Source: CAD feature listing. Evaluate the final solid. Frame: model axes, mm. A direction names the side the tool comes from. Coordinates: 2 decimals unless noted, no trailing zeros. Order: outer loops, then holes, each group sorted by start corner. A loop starts at its lowest first (then second) coordinate and runs counter-clockwise, first axis right, second up. Notation, with made-up numbers: (-30.75, 36.5) -> (13.25, 36.5) arc R30 cw to (13.25, 61.5) -> close; hole circle Ø11 at (13, 41). An arc over 180 degrees is marked (long way). Put each result on its own line as item: value.
from build123d import *

# Parameters (mm, degrees)
F0_R     = 11
F0_R_2   = 4
F1_DEPTH = 5.5
F2_R     = 12.5
F2_R_2   = 4
F3_DEPTH = 1.5
F4_R     = 9
F4_R_2   = 6
F5_DEPTH = 0.2
F6_R     = 9
F6_R_2   = 6
F7_DEPTH = 0.2
F8_R     = 0.3


with BuildPart() as f1:
    # F0 (on Front) → F1 (new body)
    with BuildSketch(Plane.XZ):
        Circle(F0_R)
        Circle(F0_R_2, mode=Mode.SUBTRACT)
    extrude(amount=F1_DEPTH)

    # F2 (on face) → F3 (join)
    with BuildSketch(Plane.XZ.offset(5.5)):
        Circle(F2_R)
        Circle(F2_R_2, mode=Mode.SUBTRACT)
    extrude(amount=F3_DEPTH)

    # F4 (on face) → F5 (cut)
    with BuildSketch(Plane(origin=(0, 0, 0), x_dir=(-1, 0, 0), z_dir=(0, 1, 0))):
        Circle(F4_R)
        Circle(F4_R_2, mode=Mode.SUBTRACT)
    extrude(amount=-F5_DEPTH, mode=Mode.SUBTRACT)

    # F6 (on face) → F7 (cut)
    with BuildSketch(Plane.XZ.offset(7)):
        Circle(F6_R)
        Circle(F6_R_2, mode=Mode.SUBTRACT)
    extrude(amount=-F7_DEPTH, mode=Mode.SUBTRACT)

    # F8
    f8_edges = [f1.edges().sort_by_distance(p)[0] for p in [
        (-12.5, -7, 0),
        (-12.5, -5.5, 0),
        (-11, 0, 0),
        (-4, -7, 0),
        (-4, 0, 0),
    ]]
    fillet(f8_edges, radius=F8_R)


solid = f1.part
1. Cut plane A-A on y = -3.75. Output: boundary loops of the cut face in (x, z), plus the area to 3 significant figures.
Numbers:
outline: circle Ø22 at (0, 0); hole circle Ø8 at (0, 0)
area: 330 mm2
2. Set-up query: faces 1 (the cylindrical face through (-0.867, -3.455, -3.905)), 2 (the flat face through (2, -6.8, -6)), 3 (the flat face through (-2, -5.5, 11)). Return all of +Z, -Z, +X, -X, +Y, -Y with unobstructed straight access to the full face (end or side cutting, diameter ignored); none if empty.
Numbers:
face 1: +Y, -Y
face 2: -Y
face 3: +Y
3. Pull-direction query (X, two-part tool) for faces 4 (the flat face through (-2, -0.2, -6)), 5 (the cylindrical face through (-2.38, -2.86, -10.74)), 6 (the flat face through (3, -7, -4)); classes: pulls with the +X half, pulls with the -X half, needs draft (parallel to the pull), parting line crosses it, or undercut.
Numbers:
face 4: undercut
face 5: parting line crosses it
face 6: needs draft
4. First-contact query: pin 1 (3 mm diameter, centred on x = 4, y = -1, fed in from -Z). Flat tip, straight axial feed; report the tip coordinate or a pass-through.
Numbers:
pin 1: stops at z = -10.71
5. Ray query, line 1 along Z through (x, y) = (0, -6.9); line 2 along Z through (x, y) = (0, -0.15); line 3 along Y through (x, z) = (11, 4). Return the intervals inside material, ascending.
Numbers:
line 1: z = -12.42 to -9, -6 to -4.08, 4.08 to 6, 9 to 12.42
line 2: z = -10.96 to -9, -6 to -4.04, 4.04 to 6, 9 to 10.96
line 3: y = -7 to -5.5
